```python
from build123d import *

# Parameters (mm, degrees)
BOSS_EXTRUDE2_DEPTH = 12.7
SKETCH2_W           = 5.08
SKETCH2_H           = 5.08
BOSS_EXTRUDE3_DEPTH = 25.4


with BuildPart() as part:
    # Sketch1 → Boss-Extrude2 (new body)
    with BuildSketch(Plane.XY):
        Polygon((0, 11.176), (0, 0), (11.176, 0), (11.176, -2.794), (13.641294118, -2.794), (13.641294118, 13.716), (-5.334, 13.716), (-5.334, 2.54), (-2.794, 2.54), (-2.794, 11.176), align=None)
    extrude(amount=BOSS_EXTRUDE2_DEPTH)

    # Sketch2 → Boss-Extrude3 (add)
    with BuildSketch(Plane(origin=(0, 13.716, 0), x_dir=(1, 0, 0), z_dir=(0, 1, 0))):
        with Locations((4.153647059, -6.35)):
            Rectangle(SKETCH2_W, SKETCH2_H)
    extrude(amount=BOSS_EXTRUDE3_DEPTH)


solid = part.part
```
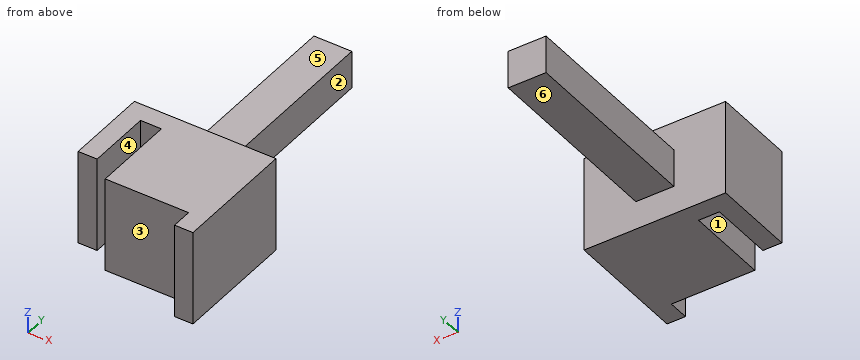
Work out the finished part from the listing and answer in its coordinate system (mm). Face numbers are marked on the shaded views. A direction names the side the tool comes from. Round coordinates to 2 decimals unless told otherwise and drop trailing zeros. Write each loop counter-clockwise with the first axis right and the second up, starting at its lowest first coordinate (ties: lowest second). Pieces come first, ordered by that corner, then holes. Notation, with made-up numbers: (78.25, -39) - (111.25, -39) arc R5 ccw to (111.25, -31) - close; hole circle Ø6 at (-15, 28). An arc over 180 degrees is marked (long way). Return JSON: item names as keys, results as strings. Group by question number.
Q1. The part is cut by section C-C on x = 2.5. Write down the section's boundary in (y, z), then the cut area to 3 significant figures.
Q2. The mould has two halves that part along X. Classify the marked faces 1, 2 and 3: released by +X, released by -X, zero draft, split by the parting line, or undercut.
Q3. The part is cut by section B-B on z = 11. Write down the section's boundary in (x, y), then the cut area to 3 significant figures.
Q4. Find the intervals of material crossed by L1, parallel to X at y = 4.5, z = 11.75; L2, parallel to Y at x = 7.25, z = 11; L3, parallel to Y at x = -2, z = 10.5, in increasing order.
Q5. For the marked faces 4, 5 and 6, determine the directions among +Z, -Z, +X, -X, +Y, -Y from which every point of the face is accessible in a straight line to the end or side of a thin tool.
Q6. The part is cut by section D-D on z = 8.5. Write down the section's boundary in (x, y).
Q7. Each of these flat-tipped pins is pushed along its axis until it touches: pin 1 Ø2 at (x, z) = (10, 7) entering from -Y; pin 2 Ø2.5 at (x, y) = (5.5, 29) entering from +Z; pin 3 Ø1.5 at (x, y) = (3.5, 20.5) entering from -Z; pin 4 Ø6 at (x, z) = (1.5, 4.5) entering from +Y. Where does it stop, or does it pass through?
Q8. The part is cut by section A-A on y = 4.5. Write down the section's boundary in (x, z), then the cut area to 3 significant figures.
Solved:
{
 "1": {"outline": "(0, 0) - (13.72, 0) - (13.72, 3.81) - (39.12, 3.81) - (39.12, 8.89) - (13.72, 8.89) - (13.72, 12.7) - (0, 12.7) - close", "area": "303 mm²"},
 "2": {"face 1": "undercut", "face 2": "released by +X", "face 3": "zero draft"},
 "3": {"outline": "(-5.33, 2.54) - (-2.79, 2.54) - (-2.79, 11.18) - (0, 11.18) - (0, 0) - (11.18, 0) - (11.18, -2.79) - (13.64, -2.79) - (13.64, 13.72) - (-5.33, 13.72) - close", "area": "229 mm²"},
 "4": {"L1": "-5.33 to -2.79, 0 to 13.64", "L2": "0 to 13.72", "L3": "11.18 to 13.72"},
 "5": {"face 4": "+Z, -Z, -Y", "face 5": "+Z, +X, -X, +Y", "face 6": "-Z, +X, -X, +Y"},
 "6": {"outline": "(-5.33, 2.54) - (-2.79, 2.54) - (-2.79, 11.18) - (0, 11.18) - (0, 0) - (11.18, 0) - (11.18, -2.79) - (13.64, -2.79) - (13.64, 13.72) - (6.69, 13.72) - (6.69, 39.12) - (1.61, 39.12) - (1.61, 13.72) - (-5.33, 13.72) - close"},
 "7": {"pin 1": "y = 0", "pin 2": "z = 8.89", "pin 3": "z = 3.81", "pin 4": "y = 39.12"},
 "8": {"outline": "(-5.33, 0) - (-2.79, 0) - (-2.79, 12.7) - (-5.33, 12.7) - close; (0, 0) - (13.64, 0) - (13.64, 12.7) - (0, 12.7) - close", "area": "206 mm²"}
}
